Part model, mm, in its own coordinate system. A direction names the side the tool comes from. Give positions to 0.01 mm unless a question says otherwise; leave off trailing zeros. Write each loop counter-clockwise with the first axis right and the second up, starting at its lowest first coordinate (ties: lowest second). Pieces come first, ordered by that corner, then holes.
from build123d import *

# Parameters (mm, degrees)
SKETCH1_W                      = 170
SKETCH1_H                      = 31.5
BOSS_EXTRUDE1_DEPTH            = 14.5
SKETCH2_W                      = 29.500000008
SKETCH2_H                      = 7.499999998
CUT_EXTRUDE1_DEPTH             = 174.50072046
CUT_EXTRUDE2_DEPTH             = 174.50072046
SKETCH4_W                      = 10.000000025
SKETCH4_H                      = 6.5
BOSS_EXTRUDE2_DEPTH            = 100
SKETCH5_W                      = 6
SKETCH5_H                      = 94
CUT_EXTRUDE3_DEPTH             = 4
SKETCH6_W                      = 11.5
SKETCH6_H                      = 75
F_12_0_12_DIAMETER_HOLE1_D     = 12
F_12_0_12_DIAMETER_HOLE1_DEPTH = 3
F_1_0_1_DIAMETER_HOLE1_D       = 1
F_1_0_1_DIAMETER_HOLE1_DEPTH   = 1
F_20_0_20_DIAMETER_HOLE1_D     = 20
F_20_0_20_DIAMETER_HOLE1_DEPTH = 79


with BuildPart() as part:
    # Sketch1 → Boss-Extrude1 (new body)
    with BuildSketch(Plane.XZ):
        with Locations((85, -15.75)):
            Rectangle(SKETCH1_W, SKETCH1_H)
    extrude(amount=-BOSS_EXTRUDE1_DEPTH)

    # Sketch2 → Cut-Extrude1 (cut, through all)
    with BuildSketch(Plane(origin=(170, 0, 0), x_dir=(0, 0, -1), z_dir=(1, 0, 0))):
        with Locations((16.749999996, 10.750000001)):
            Rectangle(SKETCH2_W, SKETCH2_H)
    extrude(amount=-CUT_EXTRUDE1_DEPTH, mode=Mode.SUBTRACT)

    # Sketch3 → Cut-Extrude2 (cut, through all)
    with BuildSketch(Plane.XY):
        with BuildLine():
            Line((160, 12.5), (10, 12.5))
            ThreePointArc((10, 12.5), (8.500000001, 11.000000001), (10, 9.500000002))
            Line((10, 9.500000002), (160, 9.500000002))
            ThreePointArc((160, 9.500000002), (161.499999999, 11.000000001), (160, 12.5))
        make_face()
    extrude(amount=-CUT_EXTRUDE2_DEPTH, mode=Mode.SUBTRACT)

    # Sketch4 → Boss-Extrude2 (add)
    with BuildSketch(Plane(origin=(0, 7.000000002, 0), x_dir=(-1, 0, 0), z_dir=(0, 1, 0))):
        with Locations((-162.500000003, -18.249999999)):
            Rectangle(SKETCH4_W, SKETCH4_H)
    extrude(amount=BOSS_EXTRUDE2_DEPTH)

    # Sketch5 → Cut-Extrude3 (cut)
    with BuildSketch(Plane.XY.offset(-14.999999999)):
        with Locations((162.5, 57)):
            Rectangle(SKETCH5_W, SKETCH5_H)
    extrude(amount=-CUT_EXTRUDE3_DEPTH, mode=Mode.SUBTRACT)

    # Sketch6 → Revolve1 (revolve)
    with BuildSketch(Plane.XY.offset(-16.5), mode=Mode.PRIVATE) as revolve1_sk:
        with Locations((20.75, 44.5)):
            Rectangle(SKETCH6_W, SKETCH6_H)
    revolve(revolve1_sk.sketch.rotate(Axis((15, 82, -16.5), (0, -1, 0)), 270), axis=Axis((15, 82, -16.5), (0, -1, 0)))

    # Ø12.0 (12) Diameter Hole1
    with Locations(Plane(origin=(0, 7.000000002, 0), x_dir=(1, 0, 0), z_dir=(0, 1, 0))):
        with Locations((85, 16.5)):
            Hole(F_12_0_12_DIAMETER_HOLE1_D / 2, depth=F_12_0_12_DIAMETER_HOLE1_DEPTH)

    # Ø1.0 (1) Diameter Hole1
    with Locations(Plane.XY.offset(-14.999999999)):
        with Locations((162.5, 105.5)):
            Hole(F_1_0_1_DIAMETER_HOLE1_D / 2, depth=F_1_0_1_DIAMETER_HOLE1_DEPTH)

    # Ø20.0 (20) Diameter Hole1
    with Locations(Plane(origin=(0, 82, 0), x_dir=(1, 0, 0), z_dir=(0, 1, 0))):
        with Locations((15, 16.5)):
            Hole(F_20_0_20_DIAMETER_HOLE1_D / 2, depth=F_20_0_20_DIAMETER_HOLE1_DEPTH)


solid = part.part
1) Flat gauge pins, fed straight in: P1, Ø0.8, axis at x = 162.5, y = 105.5, coming from the +Z side; P2, Ø5, axis at x = 163.5, y = 73, coming from the +Z side; P3, Ø2, axis at x = 162, z = -16, coming from the -Y side; P4, Ø8, axis at x = 163, y = 66.5, coming from the -Z side. Where does each tip first touch, or does it go through?
Check result:
P1: stops at z = -16
P2: stops at z = -15
P3: stops at y = 0
P4: stops at z = -21.5
2) Saw through at A-A (y = 69). Write the cut outline in (x, z).
Check result:
outline: circle Ø23 at (15, -16.5); (157.5, -21.5) - (167.5, -21.5) - (167.5, -15) - (165.5, -15) - (165.5, -19) - (159.5, -19) - (159.5, -15) - (157.5, -15) - close; hole circle Ø20 at (15, -16.5)
3) Saw through at C-C (x = 85). Write the cut outline in (y, z).
Check result:
outline: (0, -31.5) - (7, -31.5) - (7, -22.5) - (4, -22.5) - (4, -10.5) - (7, -10.5) - (7, -2) - (9.5, -2) - (9.5, 0) - (0, 0) - close; (12.5, -2) - (14.5, -2) - (14.5, 0) - (12.5, 0) - close
4) Drill centre lines: L1, parallel to Y at x = 162.5, z = -15.7; L2, parallel to X at y = 13, z = -21; L3, parallel to Z at x = 14.5, y = 64.5. Where is each one in solid material? Low to high.
Check result:
L1: y = 0 to 10, 104 to 105, 106 to 107
L2: x = 4.42 to 6.07, 23.93 to 25.58, 157.5 to 167.5
L3: z = -27.99 to -26.49, -6.51 to -5.01
5) Saw through at B-B (x = 110). Write the cut outline in (y, z).
Check result:
outline: (0, -31.5) - (7, -31.5) - (7, -2) - (9.5, -2) - (9.5, 0) - (0, 0) - close; (12.5, -2) - (14.5, -2) - (14.5, 0) - (12.5, 0) - close
6) Saw through at D-D (y = 86.5). Write the cut outline in (x, z), and give its area (3 significant figures).
Check result:
outline: (157.5, -21.5) - (167.5, -21.5) - (167.5, -15) - (165.5, -15) - (165.5, -19) - (159.5, -19) - (159.5, -15) - (157.5, -15) - close
area: 41.0 mm2
7) Mould opens along Y. For faces 1 (the flat face through (86, 9, -2)), 2 (the flat face through (163, 107, -18)), 3 (the flat face through (165.5, 56, -17)), 4 (the flat face through (162, 104, -17)) say: +Y half, -Y half, draft (parallel to the pull), parting line (faces both ways), or undercut.
Check result:
face 1: draft
face 2: +Y half
face 3: undercut
face 4: undercut
8) 3-axis set-ups, long thin cutter, end or side, ignore diameter. For faces 5 (the cylindrical face through (90.994, 5.479, -16.764)), 6 (the flat face through (163, 56, -21.5)), 7 (the flat face through (25.3, 82, -16.6)), 8 (the flat face through (162, 10, -17)): which of +Z, -Z, +X, -X, +Y, -Y reach the whole face in a straight line?
Check result:
face 5: +Y
face 6: -Z, +X, +Y
face 7: +Z, -Z, -X, +Y
face 8: none
